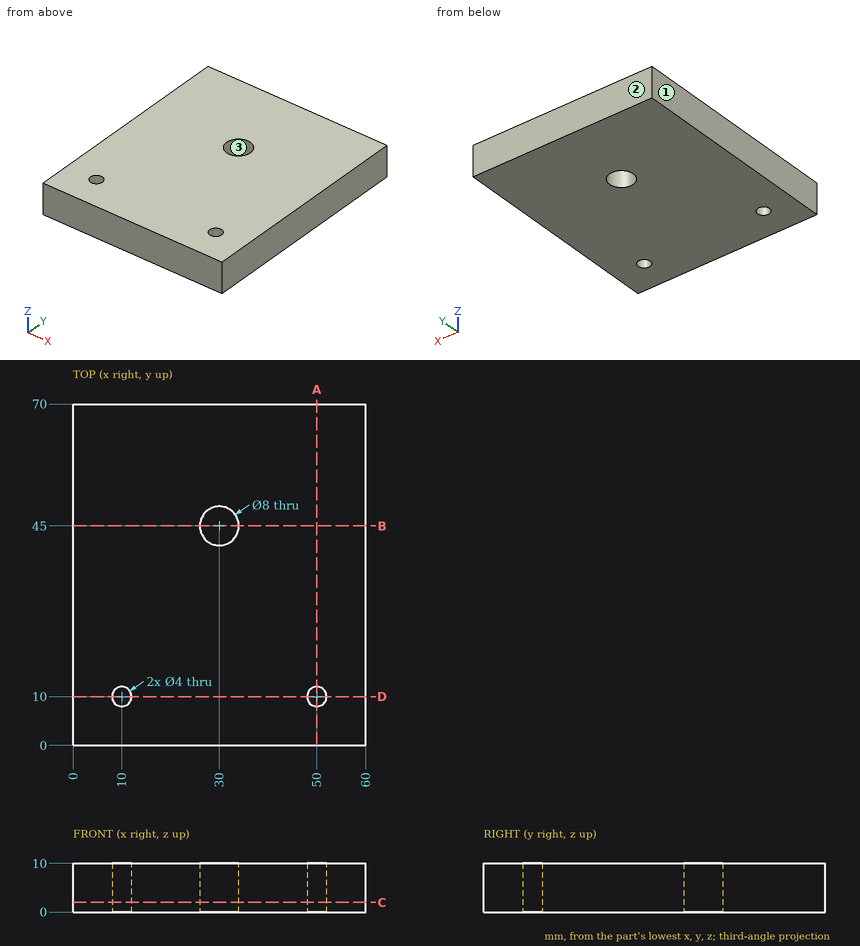
The figure shows three views and two pictorial views of one solid part (mm, origin at its lowest corner). Answer the questions. Round coordinates to 2 decimals unless told otherwise and drop trailing zeros. Write each loop counter-clockwise with the first axis right and the second up, starting at its lowest first coordinate (ties: lowest second). Pieces come first, ordered by that corner, then holes. Notation, with made-up numbers: M 82.5,88 L 132.5,88 A11 ccw 132.5,109 Z; hole C 56.25,-18 d5. An arc over 180 degrees is marked long. Write each question's results on one line, items separated by ' | '. Start each with the question number.
(1) Determine the mould class of the marked faces 1, 2 and 3 for opening direction X: +X half, -X half, draft (parallel to the pull), parting line (faces both ways), or undercut.
(2) Find the intervals of material crossed by line 1 (Y direction, x = 30, z = 7.25); line 2 (Y direction, x = 10, z = 4.75); line 3 (X direction, y = 9, z = 4.25), in increasing order.
(3) The part is cut by section B-B, the plane y = 45. Write down the section's boundary in (x, z).
(4) The part is cut by section A-A, the plane x = 50. Write down the section's boundary in (y, z).
(5) The part is cut by section C-C, the plane z = 2. Write down the section's boundary in (x, y), and give its area (3 significant figures).
(6) The part is cut by section D-D, the plane y = 10. Write down the section's boundary in (x, z), and give its area (3 significant figures).
(7) This flat-tipped pin is pushed along its axis until it touches: P1, Ø3.5, axis at x = 10, y = 10, coming from the -Z side. Where does it stop, or does it pass through?
Worked answers:
1) face 1: -X half | face 2: draft | face 3: undercut
2) line 1: y = 0 to 41, 49 to 70 | line 2: y = 0 to 8, 12 to 70 | line 3: x = 0 to 8.27, 11.73 to 48.27, 51.73 to 60
3) outline: M 0,0 L 26,0 L 26,10 L 0,10 Z; M 34,0 L 60,0 L 60,10 L 34,10 Z
4) outline: M 0,0 L 8,0 L 8,10 L 0,10 Z; M 12,0 L 70,0 L 70,10 L 12,10 Z
5) outline: M 0,0 L 60,0 L 60,70 L 0,70 Z; hole C 10,10 d4; hole C 30,45 d8; hole C 50,10 d4 | area: 4,120 mm²
6) outline: M 0,0 L 8,0 L 8,10 L 0,10 Z; M 12,0 L 48,0 L 48,10 L 12,10 Z; M 52,0 L 60,0 L 60,10 L 52,10 Z | area: 520 mm²
7) P1: passes through
